For this review, use the dimensioned drawing (mm, ordinates from the lowest corner) and the shaded views. Coordinates: 2 decimals unless noted, no trailing zeros. Loops run counter-clockwise (first coordinate to the right, second up) from the corner with the lowest first, then second, coordinate; pieces in that order, holes last. Notation, with made-up numbers: M 20,-39.5 L 71,-39.5 A11 cw 71,-29.5 Z; hole C 13,-25.75 d11. An arc over 180 degrees is marked long. One line per item, written item: value.
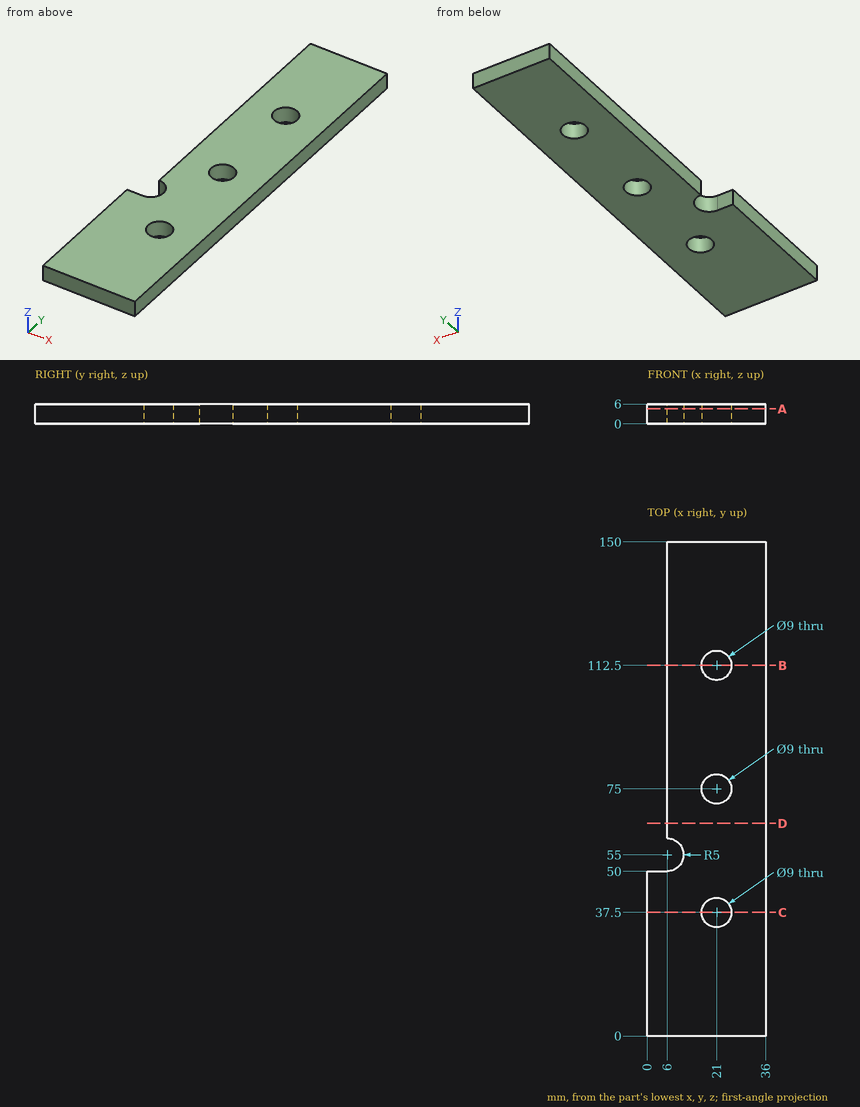
(1) Add section A-A on z = 4.55. State the section outline as (x, y) points, then the cut area to 3 significant figures.
Checks:
outline: M 0,0 L 36,0 L 36,150 L 6,150 L 6,60 A5 cw 6,50 L 0,50 Z; hole C 21,37.5 d9; hole C 21,75 d9; hole C 21,112.5 d9
area: 4,570 mm^2
(2) Add section C-C on y = 37.5. State the section outline as (x, z) points, then the cut area to 3 significant figures.
Checks:
outline: M 0,0 L 16.5,0 L 16.5,6 L 0,6 Z; M 25.5,0 L 36,0 L 36,6 L 25.5,6 Z
area: 162 mm^2
(3) Insertion check: pin 1 Ø2 at (y, z) = (133, 4.5) entering from -X. The pin has a flat end and moves straight along its axis. Give the tip position at first contact, or say it passes through.
Checks:
pin 1: x = 6
(4) Add section D-D on y = 64.5. State the section outline as (x, z) points, then the cut area to 3 significant figures.
Checks:
outline: M 6,0 L 36,0 L 36,6 L 6,6 Z
area: 180 mm^2
(5) To check wall thickness, follow L1, parallel to Y at x = 21, z = 3.25; L2, parallel to Y at x = 2, z = 4.05; L3, parallel to X at y = 55, z = 5.1. State the ranges of each line that lie inside material, in increasing order. Write a range as [from, to].
Checks:
L1: [0, 33], [42, 70.5], [79.5, 108], [117, 150]
L2: [0, 50]
L3: [11, 36]
(6) Add section B-B on y = 112.5. State the section outline as (x, z) points, then the cut area to 3 significant figures.
Checks:
outline: M 6,0 L 16.5,0 L 16.5,6 L 6,6 Z; M 25.5,0 L 36,0 L 36,6 L 25.5,6 Z
area: 126 mm^2
